The figure shows three views and two pictorial views of one solid part (mm, origin at its lowest corner). Answer the questions. A direction names the side the tool comes from. Coordinates: 2 decimals unless noted, no trailing zeros. Loops run counter-clockwise (first coordinate to the right, second up) from the corner with the lowest first, then second, coordinate; pieces in that order, holes last. Notation, with made-up numbers: (25, 3) -> (29, 3) arc R24 cw to (29, 30) -> close; hole circle Ø8 at (77.5, -17). An arc over 180 degrees is marked (long way). Use a Markdown table: item, result. Add a question column.
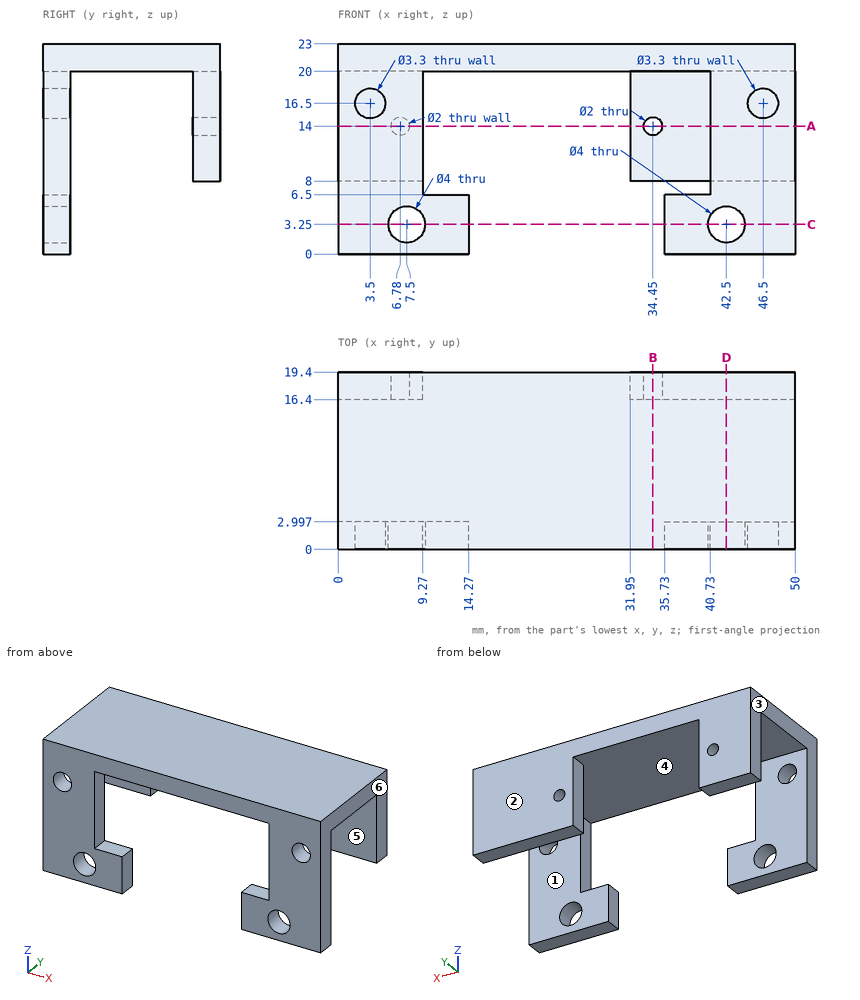
Item 1: Section A-A (z = 14) is taken. Determine the outline of the cut face in (x, y).
Item 2: Section B-B (x = 34.45) is taken. Determine the outline of the cut face in (y, z).
Item 3: For a pull along X with two mould halves and no side action, classify the marked faces 3, 4, 5 and 6 as +X half, -X half, draft (parallel to the pull), parting line (faces both ways), or undercut.
Item 4: Given pin 1 (6.5 mm diameter, centred on x = 7.5, z = 3.25, fed in from +Y); pin 2 (10 mm diameter, centred on x = 12.5, y = 11.5, fed in from -Z); pin 3 (2.5 mm diameter, centred on x = 5, y = 18, fed in from -Z), each flat-ended and moving along its own axis, determine where each tip first touches the part or whether it passes through.
Item 5: For the marked faces 1 and 2, determine the directions among +Z, -Z, +X, -X, +Y, -Y from which every point of the face is accessible in a straight line to the end or side of a thin tool.
Item 6: Section D-D (x = 42.5) is taken. Determine the outline of the cut face in (y, z).
Item 7: Section C-C (z = 3.25) is taken. Determine the outline of the cut face in (x, y).
Item 8: Find the intervals of material crossed by probe 1 along X at (y, z) = (18.75, 14); probe 2 along Z at (x, y) = (42.5, 2.3); probe 3 along X at (y, z) = (0.8, 16.5), in increasing order.
Output:
| question | item | result |
|---|---|---|
| 1 | outline | (0, 0) -> (9.27, 0) -> (9.27, 3) -> (0, 3) -> close; (0, 16.4) -> (5.78, 16.4) -> (5.78, 19.4) -> (0, 19.4) -> close; (7.78, 16.4) -> (9.27, 16.4) -> (9.27, 19.4) -> (7.78, 19.4) -> close; (31.95, 16.4) -> (33.45, 16.4) -> (33.45, 19.4) -> (31.95, 19.4) -> close; (35.45, 16.4) -> (50, 16.4) -> (50, 19.4) -> (35.45, 19.4) -> close; (40.73, 0) -> (50, 0) -> (50, 3) -> (40.73, 3) -> close |
| 2 | outline | (0, 20) -> (16.4, 20) -> (16.4, 15) -> (19.4, 15) -> (19.4, 23) -> (0, 23) -> close; (16.4, 8) -> (19.4, 8) -> (19.4, 13) -> (16.4, 13) -> close |
| 3 | face 3 | -X half |
| 3 | face 4 | undercut |
| 3 | face 5 | draft |
| 3 | face 6 | +X half |
| 4 | pin 1 | stops at y = 3 |
| 4 | pin 2 | stops at z = 20 |
| 4 | pin 3 | stops at z = 8 |
| 5 | face 1 | -Z, +X, -X |
| 5 | face 2 | +Z, -Z, +X, -X, +Y |
| 6 | outline | (0, 0) -> (3, 0) -> (3, 1.25) -> (0, 1.25) -> close; (0, 5.25) -> (3, 5.25) -> (3, 20) -> (16.4, 20) -> (16.4, 8) -> (19.4, 8) -> (19.4, 23) -> (0, 23) -> close |
| 7 | outline | (0, 0) -> (5.5, 0) -> (5.5, 3) -> (0, 3) -> close; (9.5, 0) -> (14.27, 0) -> (14.27, 3) -> (9.5, 3) -> close; (35.73, 0) -> (40.5, 0) -> (40.5, 3) -> (35.73, 3) -> close; (44.5, 0) -> (50, 0) -> (50, 3) -> (44.5, 3) -> close |
| 8 | probe 1 | x = 0 to 5.78, 7.78 to 9.27, 31.95 to 33.45, 35.45 to 50 |
| 8 | probe 2 | z = 0 to 1.25, 5.25 to 23 |
| 8 | probe 3 | x = 0 to 1.85, 5.15 to 9.27, 40.73 to 44.85, 48.15 to 50 |
